Design review of the part built by this model. Coordinates are the model's own, in mm. A direction names the side the tool comes from. Round coordinates to 2 decimals unless told otherwise and drop trailing zeros. Loops run counter-clockwise (first coordinate to the right, second up) from the corner with the lowest first, then second, coordinate; pieces in that order, holes last. Notation, with made-up numbers: (69, -26) - (108, -26) arc R18 ccw to (108, 4) - close; hole circle Ø8 at (16.5, -3). An arc over 180 degrees is marked (long way). Return JSON: item names as keys, results as strings. Group by question number.
from build123d import *

# Parameters (mm, degrees)
SKETCH1_R                                            = 17
BOSS_EXTRUDE1_DEPTH                                  = 5
SKETCH3_R                                            = 5.2
BOSS_EXTRUDE3_DEPTH                                  = 20
CSK_FOR_M4_HEX_SOCKET_COUNTERSUNK_CAP_SC_D           = 4
CSK_FOR_M4_HEX_SOCKET_COUNTERSUNK_CAP_SC_CSINK_D     = 9
CSK_FOR_M4_HEX_SOCKET_COUNTERSUNK_CAP_SC_CSINK_ANGLE = 90
M4_TAPPED_HOLE1_D                                    = 3
CHAMFER1_SIZE                                        = 0.5
FILLET1_R                                            = 0.3
FILLET2_R                                            = 0.5


with BuildPart() as part:
    # Sketch1 → Boss-Extrude1 (new body)
    with BuildSketch(Plane.XY):
        Circle(SKETCH1_R)
    extrude(amount=BOSS_EXTRUDE1_DEPTH)

    # Sketch3 → Boss-Extrude3 (add)
    with BuildSketch(Plane(origin=(0, 0, 0), x_dir=(-1, 0, 0), z_dir=(0, 0, -1))):
        Circle(SKETCH3_R)
    extrude(amount=BOSS_EXTRUDE3_DEPTH)

    # CSK for M4 Hex Socket Countersunk Cap Screw1 (through all)
    with Locations(Plane.XY.offset(5)):
        with Locations((0, 11.5), (11.5, 0), (0, -11.5), (-11.5, 0)):
            CounterSinkHole(CSK_FOR_M4_HEX_SOCKET_COUNTERSUNK_CAP_SC_D / 2, CSK_FOR_M4_HEX_SOCKET_COUNTERSUNK_CAP_SC_CSINK_D / 2, counter_sink_angle=CSK_FOR_M4_HEX_SOCKET_COUNTERSUNK_CAP_SC_CSINK_ANGLE)

    # M4 Tapped Hole1 (through all)
    with Locations(Plane.XY.offset(5)):
        with Locations((7.778174593, 7.778174593), (-7.778174593, -7.778174593), (-7.778174593, 7.778174593), (7.778174593, -7.778174593)):
            Hole(M4_TAPPED_HOLE1_D / 2)

    # Sketch9 → Revolve1 (revolve)
    with BuildSketch(Plane(origin=(0, 0, 0), x_dir=(0, 0, -1), z_dir=(1, 0, 0))):
        Polygon((-5, 6), (-39, 6), (-39, 5), (-44, 5), (-44, 4.8), (-45.1, 4.8), (-45.1, 5), (-48, 5), (-48, 0), (-5, 0), align=None)
    revolve(axis=Axis((0, 0, -20), (0, 0, 1)))

    # Chamfer1
    chamfer1_edges = [part.edges().sort_by_distance(p)[0] for p in [
        (0, -5, 48),
        (5.2, 0, -20),
    ]]
    chamfer(chamfer1_edges, length=CHAMFER1_SIZE)

    # Fillet1
    fillet1_edges = [part.edges().sort_by_distance(p)[0] for p in [
        (0, -5, 39),
    ]]
    fillet(fillet1_edges, radius=FILLET1_R)

    # Fillet2
    fillet2_edges = [part.edges().sort_by_distance(p)[0] for p in [
        (5.2, 0, 0),
        (0, -6, 5),
    ]]
    fillet(fillet2_edges, radius=FILLET2_R)


solid = part.part
Q1. For line 1 (Y direction, x = 0, z = 1.45); line 2 (X direction, y = -7, z = 4); line 3 (Z direction, x = -7.5, y = 10), list the stretches that pass through material, from the lowest coordinate up.
Q2. Add section A-A, the plane y = 11.5. State the section outline as (x, z) points, plus the area to 4 significant figures.
Q3. Insertion check: pin 1 Ø1 at (x, y) = (-13, -4) entering from +Z; pin 2 Ø8 at (x, z) = (3, 32) entering from -Y; pin 3 Ø4.5 at (x, y) = (-11.5, 0) entering from +Z; pin 4 Ø2.5 at (x, y) = (7.78, 7.78) entering from -Z. Each pin has a flat end and moves straight along its axis. Give the tip position at first contact, or say it passes through.
Q4. Tool access review of faces 1 (the flat face through (7, 0, 0)), 2 (the flat face through (7, -4, 5)), 3 (the cylindrical face through (13.1, -1.2, 1.2)): name each direction out of +Z, -Z, +X, -X, +Y, -Y from which nothing blocks a thin tool from reaching the whole face with its end or side.
Q5. Draft analysis for pull direction Y (two halves, no side actions). For faces 4 (the conical face through (13.18, -1.29, 2.62)), 5 (the flat face through (4, 4, 39)), 6 (the cylindrical face through (0, -6, 22)), state which applies: pulls with the +Y half, pulls with the -Y half, needs draft (parallel to the pull), parting line crosses it, or undercut.
Q6. Add section B-B, the plane x = 0. Give the number of separate pieces and of enclosed holes in the cut face, plus the area to 3 significant figures.
Evaluation:
{
 "1": {"line 1": "-17 to -13.5, -9.5 to 9.5, 13.5 to 17", "line 2": "-15.49 to -9.06, -6.5 to 6.5, 9.06 to 15.49", "line 3": "0 to 5"},
 "2": {"outline": "(-12.52, 0) - (-2, 0) - (-2, 2.5) - (-4.5, 5) - (-12.52, 5) - close; (2, 0) - (12.52, 0) - (12.52, 5) - (4.5, 5) - (2, 2.5) - close", "area": "98.95 mm²"},
 "3": {"pin 1": "z = 5", "pin 2": "y = -6", "pin 3": "z = 2.75", "pin 4": "through"},
 "4": {"face 1": "-Z", "face 2": "+Z", "face 3": "+Z, -Z"},
 "5": {"face 4": "undercut", "face 5": "needs draft", "face 6": "parting line crosses it"},
 "6": {"separate pieces": "3", "enclosed holes": "0", "area": "823 mm²"}
}
